```python
from build123d import *

# Parameters (mm, degrees)
EXTRUDE_THIN1_DEPTH = 60
BOSS_EXTRUDE1_DEPTH = 10
SKETCH2_R           = 60
CUT_EXTRUDE1_DEPTH  = 210.642552932
SKETCH3_W           = 74.064232883
SKETCH3_H           = 67.55464171
SKETCH3_R           = 14
CUT_EXTRUDE2_DEPTH  = 8
SKETCH3_2_R         = 14
CUT_EXTRUDE3_DEPTH  = 213.249852768
SKETCH7_R           = 4
CUT_EXTRUDE4_DEPTH  = 211.128532094


with BuildPart() as part:
    # Sketch1 → Extrude-Thin1 (new body)
    with BuildSketch(Plane.XY):
        with BuildLine():
            Line((100, 85), (-110, 85))
            Line((-110, 85), (-110, -85))
            Line((-110, -85), (100, -85))
            ThreePointArc((100, -85), (185, 0), (100, 85))
        make_face()
        with BuildLine():
            Line((100, 75), (-100, 75))
            Line((-100, 75), (-100, -75))
            Line((-100, -75), (100, -75))
            ThreePointArc((100, -75), (175, 0), (100, 75))
        make_face(mode=Mode.SUBTRACT)
    extrude(amount=-EXTRUDE_THIN1_DEPTH)

    # Sketch1<2> → Boss-Extrude1 (add)
    with BuildSketch(Plane.XY):
        with BuildLine():
            Line((-100, -75), (100, -75))
            ThreePointArc((100, -75), (175, 0), (100, 75))
            Line((100, 75), (-100, 75))
            Line((-100, 75), (-100, -75))
        make_face()
    extrude(amount=-BOSS_EXTRUDE1_DEPTH)

    # Sketch2 → Cut-Extrude1 (cut, through all)
    with BuildSketch(Plane(origin=(0, 0, -10), x_dir=(-1, 0, 0), z_dir=(0, 0, -1))):
        with Locations((-109.812010845, 0)):
            Circle(SKETCH2_R)
    extrude(amount=-CUT_EXTRUDE1_DEPTH, mode=Mode.SUBTRACT)

    # Sketch3 → Cut-Extrude2 (cut)
    with BuildSketch(Plane.XY):
        with Locations((-37.032116442, 0)):
            Rectangle(SKETCH3_W, SKETCH3_H)
        with Locations((-37.032116441, 0)):
            Circle(SKETCH3_R, mode=Mode.SUBTRACT)
    extrude(amount=-CUT_EXTRUDE2_DEPTH, mode=Mode.SUBTRACT)

    # Sketch3<2> → Cut-Extrude3 (cut, through all)
    with BuildSketch(Plane.XY):
        with Locations((-37.032116441, 0)):
            Circle(SKETCH3_2_R)
    extrude(amount=-CUT_EXTRUDE3_DEPTH, mode=Mode.SUBTRACT)

    # Sketch7 → Cut-Extrude4 (cut, through all)
    with BuildSketch(Plane.XY.offset(-8)):
        with Locations((-52.532116441, 15.5)):
            Circle(SKETCH7_R)
        with Locations((-21.532116441, 15.5)):
            Circle(SKETCH7_R)
        with Locations((-21.532116441, -15.5)):
            Circle(SKETCH7_R)
        with Locations((-52.532116441, -15.5)):
            Circle(SKETCH7_R)
    extrude(amount=-CUT_EXTRUDE4_DEPTH, mode=Mode.SUBTRACT)


solid = part.part
```
Work out the finished part from the listing and answer in its coordinate system (mm). A direction names the side the tool comes from. Give positions to 0.01 mm unless a question says otherwise; leave off trailing zeros. Write each loop counter-clockwise with the first axis right and the second up, starting at its lowest first coordinate (ties: lowest second). Pieces come first, ordered by that corner, then holes. Notation, with made-up numbers: (36.5, -39.5) -> (94.5, -39.5) arc R28 ccw to (94.5, -3.5) -> close; hole circle Ø11 at (80, 17). An arc over 180 degrees is marked (long way). Write each question's results on one line, items separated by ' | '.
1. A tool of negligible diameter and unlimited length cuts with its end or side. For faces 1 (the flat face through (-38, -33.777, -4)), 2 (the flat face through (15, -75.2, -60)), 3 (the flat face through (-1, -75, -35)), from which of +Z, -Z, +X, -X, +Y, -Y can it reach the whole face along a straight path? Write none if from no direction.
Data:
face 1: +Z | face 2: -Z, +X, -X, +Y, -Y | face 3: -Z
2. Determine the mould class of faces 4 (the flat face through (-4, 85, -30)), 5 (the cylindrical face through (184.98, -1.87, -29.58)), 6 (the flat face through (-74.064, 0, -4)) for opening direction X: +X half, -X half, draft (parallel to the pull), parting line (faces both ways), or undercut.
Data:
face 4: draft | face 5: +X half | face 6: undercut
3. Find section D-D on x = 96.5. Determine the outline of the cut face in (y, z).
Data:
outline: (-85, -60) -> (-75, -60) -> (-75, -10) -> (-58.5, -10) -> (-58.5, 0) -> (-85, 0) -> close; (58.5, -10) -> (75, -10) -> (75, -60) -> (85, -60) -> (85, 0) -> (58.5, 0) -> close
4. Find section C-C on y = 0. Determine the outline of the cut face in (x, z).
Data:
outline: (-110, -60) -> (-100, -60) -> (-100, -10) -> (-51.03, -10) -> (-51.03, -8) -> (-74.06, -8) -> (-74.06, 0) -> (-110, 0) -> close; (-23.03, -10) -> (49.81, -10) -> (49.81, 0) -> (0, 0) -> (0, -8) -> (-23.03, -8) -> close; (169.81, -10) -> (175, -10) -> (175, -60) -> (185, -60) -> (185, 0) -> (169.81, 0) -> close
5. Each of these flat-tipped pins is pushed along its axis until it touches: pin 1 Ø3 at (y, z) = (41, -39) entering from +X; pin 2 Ø10 at (x, z) = (155, -18.5) entering from -Y; pin 3 Ø2 at (x, z) = (148, -27.5) entering from -Y. Where does it stop, or does it pass through?
Data:
pin 1: x = 175.26 | pin 2: y = -68.74 | pin 3: y = -70.82
6. Find section B-B on y = -51.5. Determine the outline of the cut face in (x, z), and give its area (3 significant figures).
Data:
outline: (-110, -60) -> (-100, -60) -> (-100, -10) -> (79.03, -10) -> (79.03, 0) -> (-110, 0) -> close; (140.6, -10) -> (154.52, -10) -> (154.52, -60) -> (167.62, -60) -> (167.62, 0) -> (140.6, 0) -> close | area: 3,320 mm^2
7. Straight lines are drawn through the part: L1, parallel to X at y = 22.5, z = -2.5; L2, parallel to Y at x = 95, z = -14; L3, parallel to Z at x = 1, y = 19. For each, find the intervals that lie inside material, in ascending order.
Data:
L1: -110 to -74.06, 0 to 54.19, 165.43 to 181.97 | L2: -85 to -75, 75 to 85 | L3: -10 to 0
8. Find section A-A on z = -31. Determine the outline of the cut face in (x, y), and give its area (3 significant figures).
Data:
outline: (-110, -85) -> (100, -85) arc R85 ccw to (100, 85) -> (-110, 85) -> close; hole (-100, -75) -> (100, -75) arc R75 ccw to (100, 75) -> (-100, 75) -> close | area: 8,210 mm^2
